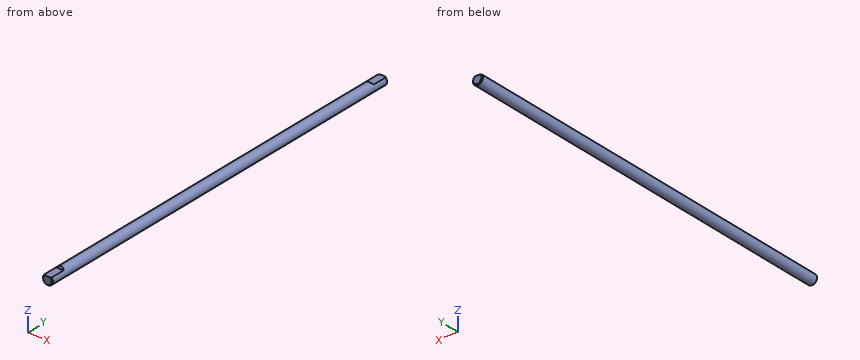
```python
from build123d import *

# Parameters (mm, degrees)
SKIZZE1_R                       = 3
AUFSATZ_LINEAR_AUSTRAGEN1_DEPTH = 240
FASE2_SIZE                      = 0.5
SCHNITT_LINEAR_START            = 2
SKIZZE2_W                       = 6
SKIZZE2_H                       = 10
SCHNITT_LINEAR_AUSTRAGEN1_DEPTH = 239.037497071
FASE1_SIZE                      = 1


with BuildPart() as part:
    # Skizze1 → Aufsatz-Linear austragen1 (new body)
    with BuildSketch(Plane(origin=(0, 0, 0), x_dir=(1, 0, 0), z_dir=(0, 1, 0))):
        with Locations(Location((0, 0, 0), (0, 0, 270))):
            Circle(SKIZZE1_R)
    extrude(amount=AUFSATZ_LINEAR_AUSTRAGEN1_DEPTH)

    # Fase2
    fase2_edges = [part.edges().sort_by_distance(p)[0] for p in [
        (0, 0, -3),
        (0, 240, -3),
    ]]
    chamfer(fase2_edges, length=FASE2_SIZE)

    # Skizze2 → Schnitt-Linear austragen1 (cut, through all)
    with BuildSketch(Plane.XY.offset(SCHNITT_LINEAR_START)):
        with Locations((0, 235)):
            Rectangle(SKIZZE2_W, SKIZZE2_H)
        with Locations((0, 5)):
            Rectangle(SKIZZE2_W, SKIZZE2_H)
    extrude(amount=SCHNITT_LINEAR_AUSTRAGEN1_DEPTH, mode=Mode.SUBTRACT)

    # Fase1
    fase1_edges = [part.edges().sort_by_distance(p)[0] for p in [
        (0, 230, 2),
        (0, 10, 2),
    ]]
    chamfer(fase1_edges, length=FASE1_SIZE - 0.0001)  # a hair under: the kernel refuses the full size


solid = part.part
```
Check sheet for the modelled part. Datum: model origin and axes. Units: mm. Give positions to 0.01 mm unless a question says otherwise; leave off trailing zeros. Order: outer loops, then holes, each group sorted by start corner. A loop starts at its lowest first (then second) coordinate and runs counter-clockwise, first axis right, second up. Notation, with made-up numbers: (62, 17.5) -> (99, 17.5) arc R16 cw to (99, 38.5) -> close; hole circle Ø3 at (-24.5, -11.5). An arc over 180 degrees is marked (long way). Return JSON: item names as keys, results as strings.
1. Cross-section at A-A, the plane y = 40.5. Record the cut outline in (x, z).
From the geometry:
{"outline": "circle Ø6 at (0, 0)"}
2. Go/stop test with flat-tipped pins: P1, Ø2, axis at x = -0.5, y = 237, coming from the +Z side; P2, Ø1.5, axis at x = -2.5, y = 199.5, coming from the -Z side. Record where each tip stops, or that it passes through.
From the geometry:
{"P1": "z = 2", "P2": "z = -2.44"}
3. Material ranges on probe 1 along Z at (x, y) = (0.5, 171); probe 2 along Z at (x, y) = (-1.7, 203); probe 3 along X at (y, z) = (99, 0.4), recorded low to high. Write a range as [from, to].
From the geometry:
{"probe 1": "[-2.96, 2.96]", "probe 2": "[-2.47, 2.47]", "probe 3": "[-2.97, 2.97]"}
